The listing builds one solid part. Answer for the finished solid, in the listing's coordinates (mm). Face numbers are marked on the shaded views. A direction names the side the tool comes from. Give positions to 0.01 mm unless a question says otherwise; leave off trailing zeros. Write each loop counter-clockwise with the first axis right and the second up, starting at its lowest first coordinate (ties: lowest second). Pieces come first, ordered by that corner, then holes.
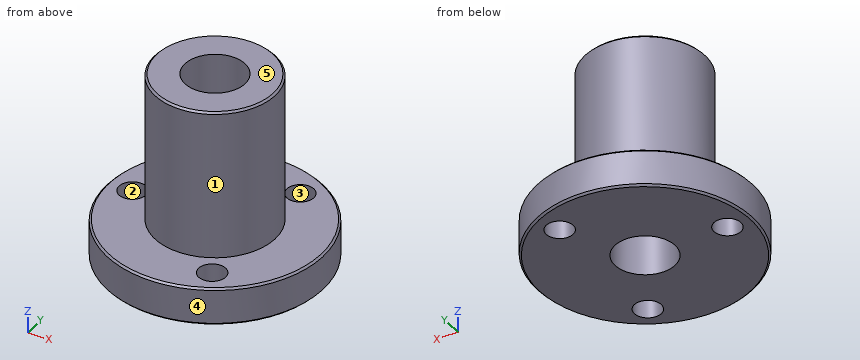
```python
from build123d import *

# Parameters (mm, degrees)
SKETCH1_W                  = 14.351
SKETCH1_H                  = 5
SKETCH2_R                  = 8.001
BOSS_EXTRUDE1_DEPTH        = 19.892
F_3_6_3_6_DIAMETER_HOLE1_D = 3.6
F_8_0_8_DIAMETER_HOLE1_D   = 8
CHAMFER1_SIZE              = 0.25


with BuildPart() as part:
    # Sketch1 → Revolve1 (revolve)
    with BuildSketch(Plane(origin=(0, 0, 0), x_dir=(1, 0, 0), z_dir=(0, 1, 0))):
        with Locations((7.1755, -2.5)):
            Rectangle(SKETCH1_W, SKETCH1_H)
    revolve(axis=Axis((0, 0, 0), (0, 0, 1)))

    # Sketch2 → Boss-Extrude1 (add)
    with BuildSketch(Plane.XY.offset(5)):
        Circle(SKETCH2_R)
    extrude(amount=BOSS_EXTRUDE1_DEPTH)

    # Ø3.6 (3.6) Diameter Hole1 (through all)
    with Locations(Plane.XY.offset(5)):
        with Locations((5.5245, -9.568714686), (-11.049, 0), (5.5245, 9.568714686)):
            Hole(F_3_6_3_6_DIAMETER_HOLE1_D / 2)

    # Ø8.0 (8) Diameter Hole1 (through all)
    with Locations(Plane.XY.offset(24.892)):
        with Locations((0, 0)):
            Hole(F_8_0_8_DIAMETER_HOLE1_D / 2)

    # Chamfer1
    chamfer1_edges = [part.edges().sort_by_distance(p)[0] for p in [
        (-14.351, 0, 5),
        (-14.351, 0, 0),
        (-8.001, 0, 24.892),
    ]]
    chamfer(chamfer1_edges, length=CHAMFER1_SIZE)


solid = part.part
```
Item 1: A cutting plane is placed at A-A, the plane x = 0. Give the vertices of the cut face in (y, z).
Conclusion:
outline: (-14.35, 0.25) - (-14.1, 0) - (-4, 0) - (-4, 24.89) - (-7.75, 24.89) - (-8, 24.64) - (-8, 5) - (-14.1, 5) - (-14.35, 4.75) - close; (4, 0) - (14.1, 0) - (14.35, 0.25) - (14.35, 4.75) - (14.1, 5) - (8, 5) - (8, 24.64) - (7.75, 24.89) - (4, 24.89) - close
Item 2: Determine the mould class of the marked faces 3, 4 and 5 for opening direction Y: pulls with the +Y half, pulls with the -Y half, needs draft (parallel to the pull), parting line crosses it, or undercut.
Conclusion:
face 3: undercut
face 4: parting line crosses it
face 5: needs draft
Item 3: Which of the six approach directions +Z, -Z, +X, -X, +Y, -Y give full straight-line access (tool end or side, diameter ignored) to the marked faces 1 and 2?
Conclusion:
face 1: +Z
face 2: +Z, -Z
Item 4: Consider probe 1 along X at (y, z) = (1.5, 4.25); probe 2 along Y at (x, z) = (5, 1.75); probe 3 along Z at (x, y) = (-9.5, 6.25). Determine where each line is inside the solid, lowest interval first.
Conclusion:
probe 1: x = -14.27 to -12.04, -10.05 to -3.71, 3.71 to 14.27
probe 2: y = -13.45 to -11.29, -7.85 to 7.85, 11.29 to 13.45
probe 3: z = 0 to 5
Item 5: A cutting plane is placed at C-C, the plane z = 12. Give the vertices of the cut face in (x, y), plus the area to 3 significant figures.
Conclusion:
outline: circle Ø16 at (0, 0); hole circle Ø8 at (0, 0)
area: 151 mm2
Item 6: A cutting plane is placed at B-B, the plane y = 0. Give the vertices of the cut face in (x, z).
Conclusion:
outline: (-14.35, 0.25) - (-14.1, 0) - (-12.85, 0) - (-12.85, 5) - (-14.1, 5) - (-14.35, 4.75) - close; (-9.25, 0) - (-4, 0) - (-4, 24.89) - (-7.75, 24.89) - (-8, 24.64) - (-8, 5) - (-9.25, 5) - close; (4, 0) - (14.1, 0) - (14.35, 0.25) - (14.35, 4.75) - (14.1, 5) - (8, 5) - (8, 24.64) - (7.75, 24.89) - (4, 24.89) - close
Item 7: Each of these flat-tipped pins is pushed along its axis until it touches: P1, Ø3, axis at x = -11.049, y = 0, coming from the +Z side; P2, Ø12, axis at x = -2.5, z = 15.5, coming from the +Y side; P3, Ø6, axis at x = 5.52, y = -9.57, coming from the +Z side; P4, Ø6, axis at y = 2, z = 11, coming from the +X side. Where does it stop, or does it pass through?
Conclusion:
P1: passes through
P2: stops at y = 8
P3: stops at z = 5
P4: stops at x = 8
